For this review, take the finished solid that the model builds, in its own axes (mm). A direction names the side the tool comes from. Round coordinates to 2 decimals unless told otherwise and drop trailing zeros. Write each loop counter-clockwise with the first axis right and the second up, starting at its lowest first coordinate (ties: lowest second). Pieces come first, ordered by that corner, then holes. Notation, with made-up numbers: (57.25, -8.75) - (111.25, -8.75) arc R20 ccw to (111.25, -4.75) - close; hole circle Ø5 at (69.25, 75.5). An arc over 180 degrees is marked (long way). Answer in a Markdown table with one row per item. Add a question column.
from build123d import *

# Parameters (mm, degrees)
EXTRUDE_THIN1_DEPTH = 20


with BuildPart() as part:
    # Sketch1 → Extrude-Thin1 (new body)
    with BuildSketch(Plane.XY):
        with BuildLine():
            Line((-38.1, 0), (-12.7, 0))
            Line((-12.7, 0), (-12.7, 12.7))
            ThreePointArc((-12.7, 12.7), (0, 25.4), (12.7, 12.7))
            Line((12.7, 12.7), (12.7, 0))
            Line((12.7, 0), (38.1, 0))
            Line((38.1, 0), (38.1, 3))
            Line((38.1, 3), (15.7, 3))
            Line((15.7, 3), (15.7, 12.7))
            ThreePointArc((15.7, 12.7), (0, 28.4), (-15.7, 12.7))
            Line((-15.7, 12.7), (-15.7, 3))
            Line((-15.7, 3), (-38.1, 3))
            Line((-38.1, 3), (-38.1, 0))
        make_face()
    extrude(amount=EXTRUDE_THIN1_DEPTH)


solid = part.part
Q1. Draft analysis for pull direction X (two halves, no side actions). For faces 1 (the face through (-38.1, 2, 10)), 2 (the face through (-14, 10, 0)), 3 (the face through (-12.7, 6, 10)), state which applies: released by +X, released by -X, zero draft, split by the parting line, or undercut.
Q2. Add section D-D on x = 24.5. State the section outline as (y, z) points.
Q3. To check wall thickness, follow probe 1 along X at (y, z) = (11.5, 14.25); probe 2 along X at (y, z) = (2.5, 6.75); probe 3 along Y at (x, z) = (-20, 4). State the ranges of each line that lie inside material, in increasing order.
Q4. Add section C-C on y = 7. State the section outline as (x, z) points, then the cut area to 3 significant figures.
Q5. Add section A-A on y = 20. State the section outline as (x, z) points, then the cut area to 3 significant figures.
Q6. Add section B-B on z = 10.5. State the section outline as (x, y) points, then the cut area to 3 significant figures.
Q7. Tool access review of faces 4 (the face through (-27, 3, 10)), 5 (the face through (-14, 10, 20)), 6 (the face through (12.7, 6, 10)), 7 (the face through (27, 3, 10)), 8 (the face through (0.345, 28.396, 9.86)): name each direction out of +Z, -Z, +X, -X, +Y, -Y from which nothing blocks a thin tool from reaching the whole face with its end or side.
Q8. Insertion check: pin 1 Ø10.5 at (y, z) = (10, 14) entering from -X; pin 2 Ø5 at (y, z) = (19.5, 9) entering from -X; pin 3 Ø10 at (x, z) = (-25, 6.5) entering from +Y. Each pin has a flat end and moves straight along its axis. Give the tip position at first contact, or say it passes through.
Answer sheet:
| question | item | result |
|---|---|---|
| 1 | face 1 | released by -X |
| 1 | face 2 | zero draft |
| 1 | face 3 | undercut |
| 2 | outline | (0, 0) - (3, 0) - (3, 20) - (0, 20) - close |
| 3 | probe 1 | x = -15.7 to -12.7, 12.7 to 15.7 |
| 3 | probe 2 | x = -38.1 to -12.7, 12.7 to 38.1 |
| 3 | probe 3 | y = 0 to 3 |
| 4 | outline | (-15.7, 0) - (-12.7, 0) - (-12.7, 20) - (-15.7, 20) - close; (12.7, 0) - (15.7, 0) - (15.7, 20) - (12.7, 20) - close |
| 4 | area | 120 mm² |
| 5 | outline | (-13.9, 0) - (-10.39, 0) - (-10.39, 20) - (-13.9, 20) - close; (10.39, 0) - (13.9, 0) - (13.9, 20) - (10.39, 20) - close |
| 5 | area | 140 mm² |
| 6 | outline | (-38.1, 0) - (-12.7, 0) - (-12.7, 12.7) arc R12.7 cw to (12.7, 12.7) - (12.7, 0) - (38.1, 0) - (38.1, 3) - (15.7, 3) - (15.7, 12.7) arc R15.7 ccw to (-15.7, 12.7) - (-15.7, 3) - (-38.1, 3) - close |
| 6 | area | 344 mm² |
| 7 | face 4 | +Z, -Z, -X, +Y |
| 7 | face 5 | +Z, +X, -X, +Y, -Y |
| 7 | face 6 | +Z, -Z, -Y |
| 7 | face 7 | +Z, -Z, +X, +Y |
| 7 | face 8 | +Z, -Z, +Y |
| 8 | pin 1 | stops at x = -15.7 |
| 8 | pin 2 | stops at x = -15.1 |
| 8 | pin 3 | stops at y = 3 |
